Geometry: final body of the model. Coordinates: model frame, mm. A direction names the side the tool comes from. Give positions to 0.01 mm unless a question says otherwise; leave off trailing zeros. Write each loop counter-clockwise with the first axis right and the second up, starting at its lowest first coordinate (ties: lowest second). Pieces come first, ordered by that corner, then holes. Notation, with made-up numbers: (39, 85) -> (82, 85) arc R32 ccw to (82, 116) -> close; hole circle Ø6 at (-12.75, -23.75). An arc over 180 degrees is marked (long way). Answer in a Markdown table with one row per item. Add a question column.
from build123d import *

# Parameters (mm, degrees)
F0_W     = 101.6
F0_H     = 50.8
F1_DEPTH = 12.7
F3_DEPTH = 25.4
F5_DEPTH = 81.28
F7_DEPTH = 125.222


with BuildPart() as f1:
    # F0 (on Top) → F1 (new body, symmetric)
    with BuildSketch(Plane.XY):
        Rectangle(F0_W, F0_H)
    extrude(amount=F1_DEPTH, both=True)

    # F2 (on face) → F3 (cut)
    with BuildSketch(Plane.XY.offset(12.7)):
        Polygon((-13.8203132717, 0), (-16.6731197387, -7.3403669521), (-9.9523638651, -9.9523638651), align=None)
        Polygon((-16.6731197387, 7.3403669521), (-13.8203132717, 0), (-9.9523638651, 9.9523638651), align=None)
        Polygon((-9.9523638651, 9.9523638651), (-13.8203132717, 0), (-9.9523638651, -9.9523638651), (0, -13.8203132717), (9.9523638651, -9.9523638651), (13.8203132717, 0), (9.9523638651, 9.9523638651), (0, 13.8203132717), align=None)
        Polygon((0, -13.8203132717), (-9.9523638651, -9.9523638651), (-7.3403669521, -16.6731197387), align=None)
        Polygon((-7.3403669521, 16.6731197387), (-9.9523638651, 9.9523638651), (0, 13.8203132717), align=None)
        Polygon((9.9523638651, -9.9523638651), (0, -13.8203132717), (7.3403669521, -16.6731197387), align=None)
        Polygon((7.3403669521, 16.6731197387), (0, 13.8203132717), (9.9523638651, 9.9523638651), align=None)
        Polygon((13.8203132717, 0), (9.9523638651, -9.9523638651), (16.6731197387, -7.3403669521), align=None)
        Polygon((16.6731197387, 7.3403669521), (9.9523638651, 9.9523638651), (13.8203132717, 0), align=None)
    extrude(amount=-F3_DEPTH, mode=Mode.SUBTRACT)

    # F4 (on face) → F5 (cut)
    with BuildSketch(Plane.XZ.offset(25.4)):
        Polygon((-7.2104095505, 0), (-8.7035782635, -3.5653209779), (-5.0820355483, -5.0820355483), align=None)
        Polygon((-8.7035782635, 3.5653209779), (-7.2104095505, 0), (-5.0820355483, 5.0820355483), align=None)
        Polygon((-5.0820355483, 5.0820355483), (-7.2104095505, 0), (-5.0820355483, -5.0820355483), (0, -7.2104095505), (5.0820355483, -5.0820355483), (7.2104095505, 0), (5.0820355483, 5.0820355483), (0, 7.2104095505), align=None)
        Polygon((0, -7.2104095505), (-5.0820355483, -5.0820355483), (-3.5653209779, -8.7035782635), align=None)
        Polygon((-3.5653209779, 8.7035782635), (-5.0820355483, 5.0820355483), (0, 7.2104095505), align=None)
        Polygon((5.0820355483, -5.0820355483), (0, -7.2104095505), (3.5653209779, -8.7035782635), align=None)
        Polygon((3.5653209779, 8.7035782635), (0, 7.2104095505), (5.0820355483, 5.0820355483), align=None)
        Polygon((7.2104095505, 0), (5.0820355483, -5.0820355483), (8.7035782635, -3.5653209779), align=None)
        Polygon((8.7035782635, 3.5653209779), (5.0820355483, 5.0820355483), (7.2104095505, 0), align=None)
    extrude(amount=-F5_DEPTH, mode=Mode.SUBTRACT)

    # F6 (on face) → F7 (cut)
    with BuildSketch(Plane.YZ.offset(50.8)):
        Polygon((-8.4402397494, 0), (-10.1716518402, -3.7750459742), (-5.7863499024, -5.7863499024), align=None)
        Polygon((-10.1716518402, 3.7750459742), (-8.4402397494, 0), (-5.7863499024, 5.7863499024), align=None)
        Polygon((-5.7863499024, 5.7863499024), (-8.4402397494, 0), (-5.7863499024, -5.7863499024), (0, -8.4402397494), (5.7863499024, -5.7863499024), (8.4402397494, 0), (5.7863499024, 5.7863499024), (0, 8.4402397494), align=None)
        Polygon((0, -8.4402397494), (-5.7863499024, -5.7863499024), (-3.7750459742, -10.1716518402), align=None)
        Polygon((-3.7750459742, 10.1716518402), (-5.7863499024, 5.7863499024), (0, 8.4402397494), align=None)
        Polygon((5.7863499024, -5.7863499024), (0, -8.4402397494), (3.7750459742, -10.1716518402), align=None)
        Polygon((3.7750459742, 10.1716518402), (0, 8.4402397494), (5.7863499024, 5.7863499024), align=None)
        Polygon((8.4402397494, 0), (5.7863499024, -5.7863499024), (10.1716518402, -3.7750459742), align=None)
        Polygon((10.1716518402, 3.7750459742), (5.7863499024, 5.7863499024), (8.4402397494, 0), align=None)
    extrude(amount=-F7_DEPTH, mode=Mode.SUBTRACT)


solid = f1.part
Q1. Line query: probe 1 along Y at (x, z) = (36, -9); probe 2 along X at (y, z) = (18, 2.5); probe 3 along X at (y, z) = (-20.5, -7.25). Output: solid intervals per line, ascending. Write a range as from..to.
Q2. Contact query for a flat-ended pin moving along its axis: pin 1 Ø4 at (x, z) = (-7.5, -2) entering from -Y. Output: stop coordinate, or through.
Q3. Section B-B on z = 1.5. Return loops of the section in (x, y).
Q4. Section C-C on y = -19. Return loops of the section in (x, z).
Q5. Access query for faces 1 (the flat face through (7.97, -20.73, -1.81)), 2 (the flat face through (4.43, -15.54, -9.31)), 3 (the flat face through (33.292, -4.795, -7.948)), 4 (the flat face through (-1, 25.4, 9)). Directions: +Z, -Z, +X, -X, +Y, -Y. A direction counts if a zero-diameter tool reaches every point of the face in a straight line with its end or side. Return the directions, or none.
Q6. Pull-direction query (Z, two-part tool) for faces 5 (the flat face through (-32.795, -4.795, -7.948)), 6 (the flat face through (-11.438, 9.375, 0.046)); classes: +Z half, -Z half, draft (parallel to the pull), parting line (faces both ways), or undercut.
Q7. Section A-A on x = 20.5. Return loops of the section in (y, z).
Q8. Section D-D on x = -2. Return loops of the section in (y, z), and give its area (3 significant figures).
Checks:
| question | item | result |
|---|---|---|
| 1 | probe 1 | -25.4..-4.31, -1.22..1.22, 4.31..25.4 |
| 1 | probe 2 | -50.8..-8.26, 8.26..50.8 |
| 1 | probe 3 | -50.8..-4.17, -0.09..0.09, 4.17..50.8 |
| 2 | pin 1 | y = -25.4 |
| 3 | outline | (-50.8, -25.4) -> (-7.84, -25.4) -> (-7.84, -15.39) -> (-9.95, -9.95) -> (-12.07, -9.13) -> (-50.8, -9.13) -> close; (-50.8, 9.13) -> (-12.07, 9.13) -> (-9.95, 9.95) -> (-7.84, 15.39) -> (-7.84, 25.4) -> (-50.8, 25.4) -> close; (7.84, -25.4) -> (50.8, -25.4) -> (50.8, -9.13) -> (12.07, -9.13) -> (9.95, -9.95) -> (7.84, -15.39) -> close; (7.84, 15.39) -> (9.95, 9.95) -> (12.07, 9.13) -> (50.8, 9.13) -> (50.8, 25.4) -> (7.84, 25.4) -> close |
| 4 | outline | (-50.8, -12.7) -> (50.8, -12.7) -> (50.8, 12.7) -> (-50.8, 12.7) -> close; hole (-8.7, -3.57) -> (-5.08, -5.08) -> (-3.57, -8.7) -> (0, -7.21) -> (3.57, -8.7) -> (5.08, -5.08) -> (8.7, -3.57) -> (7.21, 0) -> (8.7, 3.57) -> (5.08, 5.08) -> (3.57, 8.7) -> (0, 7.21) -> (-3.57, 8.7) -> (-5.08, 5.08) -> (-8.7, 3.57) -> (-7.21, 0) -> close |
| 5 | face 1 | +Y, -Y |
| 5 | face 2 | +Z, -Z |
| 5 | face 3 | +X, -X |
| 5 | face 4 | +Z, -Z, +X, -X, +Y |
| 6 | face 5 | undercut |
| 6 | face 6 | draft |
| 7 | outline | (-25.4, -12.7) -> (25.4, -12.7) -> (25.4, 12.7) -> (-25.4, 12.7) -> close; hole (-10.17, -3.78) -> (-5.79, -5.79) -> (-3.78, -10.17) -> (0, -8.44) -> (3.78, -10.17) -> (5.79, -5.79) -> (10.17, -3.78) -> (8.44, 0) -> (10.17, 3.78) -> (5.79, 5.79) -> (3.78, 10.17) -> (0, 8.44) -> (-3.78, 10.17) -> (-5.79, 5.79) -> (-10.17, 3.78) -> (-8.44, 0) -> close |
| 8 | outline | (-25.4, -12.7) -> (-14.6, -12.7) -> (-14.6, -8.05) -> (-25.4, -8.05) -> close; (-25.4, 8.05) -> (-14.6, 8.05) -> (-14.6, 12.7) -> (-25.4, 12.7) -> close; (14.6, -12.7) -> (25.4, -12.7) -> (25.4, -8.05) -> (14.6, -8.05) -> close; (14.6, 8.05) -> (25.4, 8.05) -> (25.4, 12.7) -> (14.6, 12.7) -> close |
| 8 | area | 201 mm^2 |
